from build123d import *

# Parameters (mm, degrees)
SKETCH1_W                    = 100
SKETCH1_H                    = 100
BOSS_EXTRUDE1_DEPTH          = 30
CUT_EXTRUDE1_DEPTH           = 25
SKETCH3_W                    = 20
SKETCH3_H                    = 5
CUT_EXTRUDE_THIN1_DEPTH      = 2
CUT_EXTRUDE_THIN2_DEPTH      = 1
CUT_EXTRUDE_THIN2_DEPTH_BACK = 3


with BuildPart() as part:
    # Sketch1 → Boss-Extrude1 (new body)
    with BuildSketch(Plane(origin=(0, 0, 0), x_dir=(1, 0, 0), z_dir=(0, 1, 0))):
        Rectangle(SKETCH1_W, SKETCH1_H)
    extrude(amount=BOSS_EXTRUDE1_DEPTH)

    # Sketch2 → Cut-Extrude1 (cut)
    with BuildSketch(Plane(origin=(0, 30, 0), x_dir=(1, 0, 0), z_dir=(0, 1, 0))):
        Polygon((30, 10), (10, 30), (-10, 30), (-30, 10), (-30, -10), (-10, -30), (10, -30), (30, -10), align=None)
    extrude(amount=-CUT_EXTRUDE1_DEPTH, mode=Mode.SUBTRACT)

    # Sketch3 → Cut-Extrude-Thin1 (cut)
    with BuildSketch(Plane(origin=(0, 30, 0), x_dir=(1, 0, 0), z_dir=(0, 1, 0))):
        with Locations((0, 38)):
            Rectangle(SKETCH3_W, SKETCH3_H)
    extrude(amount=-CUT_EXTRUDE_THIN1_DEPTH, mode=Mode.SUBTRACT)

    # Sketch4 → Cut-Extrude-Thin2 (cut, two sides)
    with BuildSketch(Plane(origin=(0, 30, 0), x_dir=(1, 0, 0), z_dir=(0, 1, 0))) as cut_extrude_thin2_sk:
        Polygon((51.767766953, -48.232233047), (34.090097423, -30.554563517), (30.554563517, -34.090097423), (48.232233047, -51.767766953), align=None)
    extrude(amount=CUT_EXTRUDE_THIN2_DEPTH, mode=Mode.SUBTRACT)
    extrude(cut_extrude_thin2_sk.sketch, amount=-CUT_EXTRUDE_THIN2_DEPTH_BACK, mode=Mode.SUBTRACT)


solid = part.part
Design review of the part built by this model. Coordinates are the model's own, in mm. A direction names the side the tool comes from. Coordinates: 2 decimals unless noted, no trailing zeros. Order: outer loops, then holes, each group sorted by start corner. A loop starts at its lowest first (then second) coordinate and runs counter-clockwise, first axis right, second up. Notation, with made-up numbers: M -31,76 L 3,76 A23 cw 3,109 Z; hole C 78,-34.75 d10. An arc over 180 degrees is marked long. Use a Markdown table: item, result.
(1) Add section C-C (x = -2.5). Give the boundary of the cut face in (y, z), then the cut area to 3 significant figures.
Worked answers:
| item | result |
|---|---|
| outline | M 0,-50 L 30,-50 L 30,-40.5 L 28,-40.5 L 28,-35.5 L 30,-35.5 L 30,-30 L 5,-30 L 5,30 L 30,30 L 30,50 L 0,50 Z |
| area | 1,490 mm2 |
(2) Add section A-A (y = 14). Give the boundary of the cut face in (x, z).
Worked answers:
| item | result |
|---|---|
| outline | M -50,-50 L 50,-50 L 50,50 L -50,50 Z; hole M -30,-10 L -10,-30 L 10,-30 L 30,-10 L 30,10 L 10,30 L -10,30 L -30,10 Z |
(3) For P1, Ø2.5, axis at x = 3.5, z = -37, coming from the +Y side; P2, Ø6, axis at x = 25, z = 1.5, coming from the +Y side, all flat-tipped, find the tip position at first contact; note any pin that passes through.
Worked answers:
| item | result |
|---|---|
| P1 | stops at y = 28 |
| P2 | stops at y = 5 |
(4) Wall thickness on probe 1 along X at (y, z) = (24.75, -7); probe 2 along X at (y, z) = (28.75, -37); probe 3 along Y at (x, z) = (29.5, 0.5): over which ranges is each line inside the solid? List them lowest first.
Worked answers:
| item | result |
|---|---|
| probe 1 | x = -50 to -30, 30 to 50 |
| probe 2 | x = -50 to -10, 10 to 50 |
| probe 3 | y = 0 to 5 |
(5) Add section B-B (z = 3). Give the boundary of the cut face in (x, y).
Worked answers:
| item | result |
|---|---|
| outline | M -50,0 L 50,0 L 50,30 L 30,30 L 30,5 L -30,5 L -30,30 L -50,30 Z |
(6) For faces 1 (the flat face through (42.156, 28.521, 38.621)), 2 (the flat face through (-23, 30, -23)), list the 3-axis set-ups (+Z, -Z, +X, -X, +Y, -Y) from which the entire face can be reached by the end or side of a thin tool; tool diameter is ignored.
Worked answers:
| item | result |
|---|---|
| face 1 | +Y |
| face 2 | +Z, -Z, +X, -X, +Y |
(7) Add section D-D (z = -26.5). Give the boundary of the cut face in (x, y), then the cut area to 4 significant figures.
Worked answers:
| item | result |
|---|---|
| outline | M -50,0 L 50,0 L 50,30 L 13.5,30 L 13.5,5 L -13.5,5 L -13.5,30 L -50,30 Z |
| area | 2,325 mm2 |
(8) Draft analysis for pull direction X (two halves, no side actions). For faces 3 (the flat face through (-50, 15, 1)), 4 (the flat face through (20, 18, 20)), 5 (the flat face through (-30, 18, 0)), 6 (the flat face through (-1, 0, -1)), state which applies: released by +X, released by -X, zero draft, split by the parting line, or undercut.
Worked answers:
| item | result |
|---|---|
| face 3 | released by -X |
| face 4 | undercut |
| face 5 | undercut |
| face 6 | zero draft |
